CAD build for the part. Positions are in the model's coordinates, mm. A direction names the side the tool comes from. Round coordinates to 2 decimals unless told otherwise and drop trailing zeros. Loops run counter-clockwise (first coordinate to the right, second up) from the corner with the lowest first, then second, coordinate; pieces in that order, holes last.
from build123d import *

# Parameters (mm, degrees)
SKETCH1_W           = 26.5
SKETCH1_H           = 20
BOSS_EXTRUDE1_DEPTH = 8.6
SKETCH2_W           = 6.5
SKETCH2_H           = 6.5
BOSS_EXTRUDE2_DEPTH = 1.5


with BuildPart() as part:
    # Sketch1 → Boss-Extrude1 (new body)
    with BuildSketch(Plane(origin=(0, 0, 0), x_dir=(1, 0, 0), z_dir=(0, 1, 0))):
        Rectangle(SKETCH1_W, SKETCH1_H)
    extrude(amount=BOSS_EXTRUDE1_DEPTH)

    # Sketch2 → Boss-Extrude2 (add)
    with BuildSketch(Plane(origin=(13.25, 0, 0), x_dir=(0, 0, -1), z_dir=(1, 0, 0))):
        with Locations((5.75, 5.35)):
            Rectangle(SKETCH2_W, SKETCH2_H)
    extrude(amount=BOSS_EXTRUDE2_DEPTH)

    # Sketch6 → Revolve1 (revolve)
    with BuildSketch(Plane.XY.offset(-5.75), mode=Mode.PRIVATE) as revolve1_sk:
        Polygon((14.75, 5.35), (14.75, 2.7), (17.75, 2.7), (17.75, 0.85), (26.25, 0.85), (26.25, 2.05), (36.25, 2.05), (36.25, 2.55), (39.25, 2.55), (39.25, 2.85), (44.65, 2.85), (44.65, 3.35), (52.05, 3.35), (52.05, -2.65), (54.05, -2.65), (54.05, 3.6), (65.05, 3.6), (65.05, -6.15), (72.05, -6.15), (72.05, 5.35), align=None)
    revolve(revolve1_sk.sketch.rotate(Axis((14.75, 5.35, -5.75), (1, 0, 0)), 270), axis=Axis((14.75, 5.35, -5.75), (1, 0, 0)))


solid = part.part
Item 1: Cut at B-B (x = 35). List the corners of the cut face in (y, z), plus the area to 3 significant figures.
Verdict:
outline: circle Ø6.6 at (5.35, -5.75)
area: 34.2 mm2
Item 2: Cut at C-C (y = -4.25). List the corners of the cut face in (x, z), plus the area to 3 significant figures.
Verdict:
outline: (65.05, -12.08) - (72.05, -12.08) - (72.05, 0.58) - (65.05, 0.58) - close
area: 88.6 mm2
Item 3: Mould opens along X. For faces 5 (the cylindrical face through (37.771, 7.834, -4.458)), 6 (the flat face through (0, 4, -10)), 7 (the flat face through (72.05, 5, -6)) say: released by +X, released by -X, zero draft, split by the parting line, or undercut.
Verdict:
face 5: undercut
face 6: zero draft
face 7: released by +X
Item 4: 3-axis set-ups, long thin cutter, end or side, ignore diameter. For faces 1 (the flat face through (-13.25, 4, 0)), 2 (the flat face through (14, 5, -9)), 3 (the cylindrical face through (16.27, 2.72, -6.09)), 4 (the flat face through (1, 8.6, 0)): which of +Z, -Z, +X, -X, +Y, -Y reach the whole face in a straight line?
Verdict:
face 1: +Z, -Z, -X, +Y, -Y
face 2: -Z, +Y, -Y
face 3: none
face 4: +Z, -Z, -X, +Y
Item 5: Flat gauge pins, fed straight in: P1, Ø6, axis at x = 2.5, z = -1.5, coming from the -Y side; P2, Ø0.8, axis at x = 14, y = 4, coming from the +Z side; P3, Ø2.5, axis at x = 3, y = 4.5, coming from the -Z side. Where does each tip first touch, or does it go through?
Verdict:
P1: stops at y = 0
P2: stops at z = -2.5
P3: stops at z = -10
Item 6: Wall check: L1, parallel to X at y = 2.5, z = 1.25; L2, parallel to X at y = 3.5, z = -1.75; L3, parallel to X at y = 13, z = -6. Give the ranges that are in metal, low to high.
Verdict:
L1: x = -13.25 to 13.25, 52.05 to 54.05, 65.05 to 72.05
L2: x = -13.25 to 13.25, 17.75 to 26.25, 52.05 to 54.05, 65.05 to 72.05
L3: x = 52.05 to 54.05, 65.05 to 72.05
Item 7: Cut at D-D (x = 5). List the corners of the cut face in (y, z).
Verdict:
outline: (0, -10) - (8.6, -10) - (8.6, 10) - (0, 10) - close
Item 8: Cut at A-A (z = 1). List the corners of the cut face in (x, y), plus the area to 3 significant figures.
Verdict:
outline: (-13.25, 0) - (13.25, 0) - (13.25, 8.6) - (-13.25, 8.6) - close; (52.05, 1.06) - (54.05, 1.06) - (54.05, 9.64) - (52.05, 9.64) - close; (65.05, -3.96) - (72.05, -3.96) - (72.05, 14.66) - (65.05, 14.66) - close
area: 375 mm2
